The drawing under review shows one solid part. Ordinate dimensions are in mm from its lowest x, y, z. Give positions to 0.01 mm unless a question says otherwise; leave off trailing zeros. Order: outer loops, then holes, each group sorted by start corner. A loop starts at its lowest first (then second) coordinate and runs counter-clockwise, first axis right, second up. Notation, with made-up numbers: (70, 24.25) - (85, 24.25) arc R12 ccw to (85, 33.25) - close; hole circle Ø10 at (58, -30.5). An arc over 180 degrees is marked (long way). Use CSV: the item, a comma, the result in double quotes. Start each with the question number.
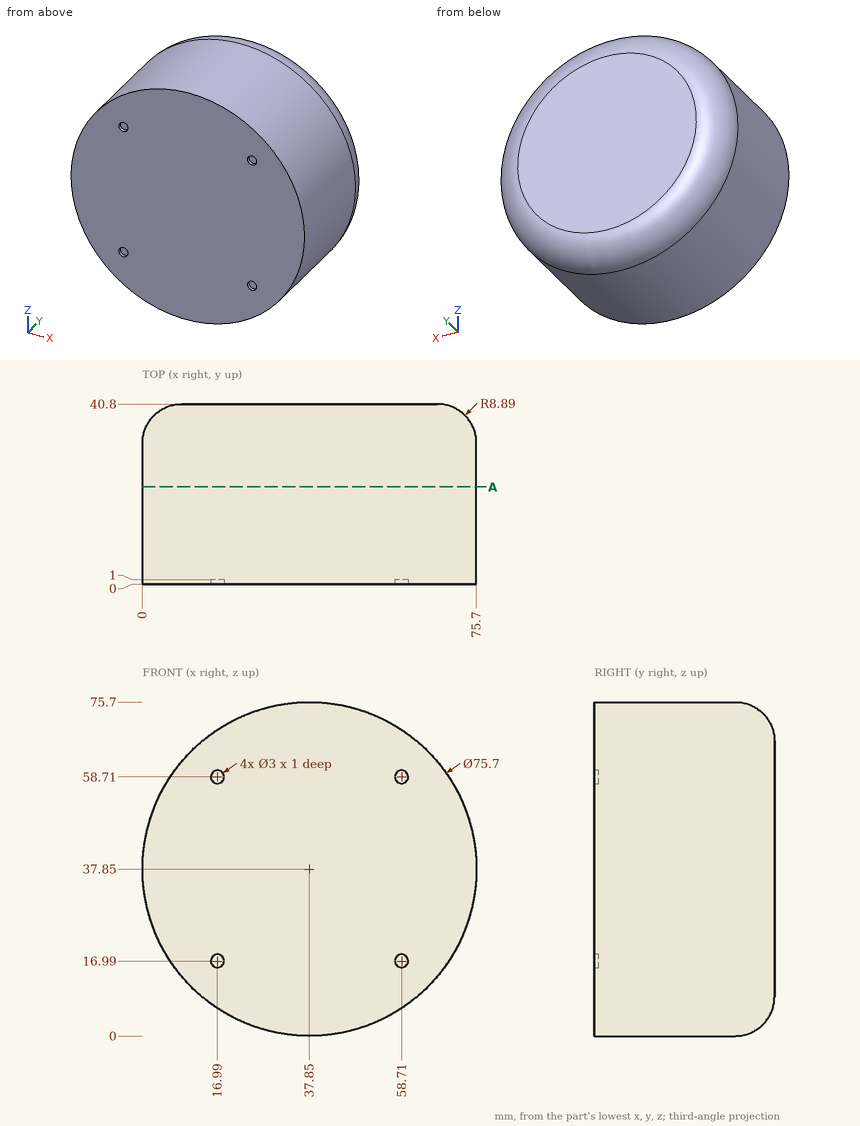
1. To check wall thickness, follow L1, parallel to Y at x = 67, z = 41; L2, parallel to X at y = 35.5, z = 51.5; L3, parallel to Z at x = 49, y = 7. State the ranges of each line that lie inside material, in increasing order. Write a range as [from, to].
2. Clearance check with flat-ended pins moving along their axes: pin 1 (1 mm diameter, centred on y = 32, z = 64, fed in from -X); pin 2 (3 mm diameter, centred on y = 30.5, z = 39.5, fed in from -X); pin 3 (6 mm diameter, centred on x = 68, z = 14, fed in from +Y). State where each tip first meets the part, or that it passes through.
3. Consider section A-A (y = 22). Give the boundary of the cut face in (x, z), and give its area (3 significant figures).
Answers follow:
1,L1,"y = [0, 40.79]"
1,L2,"x = [3.36, 72.34]"
1,L3,"z = [1.68, 74.02]"
2,pin 1,"stops at x = 10.02"
2,pin 2,"stops at x = 0"
2,pin 3,"stops at y = 37.99"
3,outline,"circle Ø75.7 at (37.85, 37.85)"
3,area,"4,500 mm^2"
